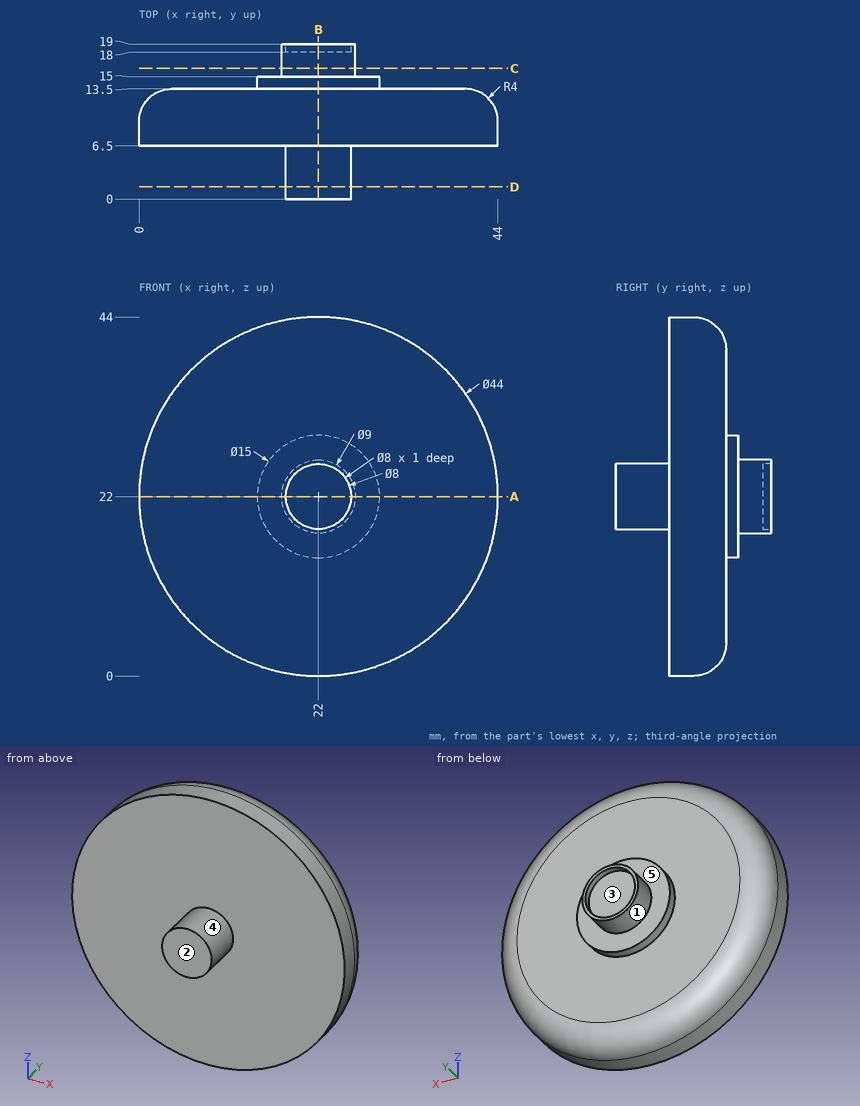
Design review of the part shown in the three views and the two pictorial views. Dimensions are in mm from the part's minimum x, y and z. A direction names the side the tool comes from. Round coordinates to 2 decimals unless told otherwise and drop trailing zeros. Loops run counter-clockwise (first coordinate to the right, second up) from the corner with the lowest first, then second, coordinate; pieces in that order, holes last. Notation, with made-up numbers: (8, -8) -> (54, -8) arc R24 ccw to (54, 17) -> close; hole circle Ø9 at (-37, -11.5). An arc over 180 degrees is marked (long way). Return JSON: item names as keys, results as strings.
(1) Add section B-B on x = 22. Write out the cut boundary in (y, z).
Solved:
{"outline": "(0, 18) -> (6.5, 18) -> (6.5, 0) -> (9.5, 0) arc R4 ccw to (13.5, 4) -> (13.5, 14.5) -> (15, 14.5) -> (15, 17.5) -> (19, 17.5) -> (19, 18) -> (18, 18) -> (18, 26) -> (19, 26) -> (19, 26.5) -> (15, 26.5) -> (15, 29.5) -> (13.5, 29.5) -> (13.5, 40) arc R4 ccw to (9.5, 44) -> (6.5, 44) -> (6.5, 26) -> (0, 26) -> close"}
(2) For line 1 (X direction, y = 18.35, z = 22); line 2 (Y direction, x = 14.5, z = 21); line 3 (Y direction, x = 17, z = 22.5), list the stretches that pass through material, from the lowest coordinate up.
Solved:
{"line 1": "17.5 to 18, 26 to 26.5", "line 2": "6.5 to 13.5", "line 3": "6.5 to 15"}
(3) For the marked faces 4 and 5, list the 3-axis set-ups (+Z, -Z, +X, -X, +Y, -Y) from which the entire face can be reached by the end or side of a thin tool; tool diameter is ignored.
Solved:
{"face 4": "-Y", "face 5": "+Y"}
(4) Add section D-D on y = 1.5. Write out the cut boundary in (x, z).
Solved:
{"outline": "circle Ø8 at (22, 22)"}
(5) Add section A-A on z = 22. Write out the cut boundary in (x, y), plus the area to 3 significant figures.
Solved:
{"outline": "(0, 6.5) -> (18, 6.5) -> (18, 0) -> (26, 0) -> (26, 6.5) -> (44, 6.5) -> (44, 9.5) arc R4 ccw to (40, 13.5) -> (29.5, 13.5) -> (29.5, 15) -> (26.5, 15) -> (26.5, 19) -> (26, 19) -> (26, 18) -> (18, 18) -> (18, 19) -> (17.5, 19) -> (17.5, 15) -> (14.5, 15) -> (14.5, 13.5) -> (4, 13.5) arc R4 ccw to (0, 9.5) -> close", "area": "404 mm2"}
(6) The part is to be moulded in two halves that separate along Z. For the marked faces 1, 2 and 3, say which applies: released by +Z, released by -Z, zero draft, split by the parting line, or undercut.
Solved:
{"face 1": "split by the parting line", "face 2": "zero draft", "face 3": "undercut"}
(7) For pin 1 (10 mm diameter, centred on x = 38.5, z = 18.5, fed in from -Y); pin 2 (5 mm diameter, centred on x = 16, z = 10.5, fed in from +Y); pin 3 (1.5 mm diameter, centred on x = 35.5, y = 9.5, fed in from +Z), all flat-tipped, find the tip position at first contact; note any pin that passes through.
Solved:
{"pin 1": "y = 6.5", "pin 2": "y = 13.5", "pin 3": "z = 39.93"}
(8) Add section C-C on y = 16. Write out the cut boundary in (x, z).
Solved:
{"outline": "circle Ø9 at (22, 22)"}
